Here's how the part is built. I have some questions about the finished solid (model axes, mm). Round coordinates to 2 decimals unless told otherwise and drop trailing zeros. Write each loop counter-clockwise with the first axis right and the second up, starting at its lowest first coordinate (ties: lowest second). Pieces come first, ordered by that corner, then holes. Notation, with made-up numbers: (30.25, 56.25) -> (81.25, 56.25) arc R32 ccw to (81.25, 86.25) -> close; hole circle Ø5 at (6.5, 57.25). An arc over 180 degrees is marked (long way). Answer as CSV lines item,"result".
from build123d import *

# Parameters (mm, degrees)
SKETCH001_W      = 8.45
SKETCH001_H      = 8.45
EXTRUDE001_DEPTH = 3
SKETCH_W         = 148.3
SKETCH_H         = 12.45
SKETCH_W_2       = 8.45
SKETCH_H_2       = 8.45
EXTRUDE_DEPTH    = 6.8


with BuildPart() as extrude001:
    # Sketch001 → Extrude001 (new body)
    with BuildSketch(Plane.XY):
        with Locations((-142.725, 0)):
            Rectangle(SKETCH001_W, SKETCH001_H)
        with Locations((7.5, 0)):
            Rectangle(SKETCH001_W, SKETCH001_H)
    extrude(amount=EXTRUDE001_DEPTH)


with BuildPart() as cut:
    # Sketch → Extrude (new body)
    with BuildSketch(Plane.XY):
        with Locations((-67.925, 0)):
            Rectangle(SKETCH_W, SKETCH_H)
        Rectangle(SKETCH_W_2, SKETCH_H_2, mode=Mode.SUBTRACT)
        with Locations((-10.45, 0)):
            Rectangle(SKETCH_W_2, SKETCH_H_2, mode=Mode.SUBTRACT)
        with Locations((-20.9, 0)):
            Rectangle(SKETCH_W_2, SKETCH_H_2, mode=Mode.SUBTRACT)
        with Locations((-31.35, 0)):
            Rectangle(SKETCH_W_2, SKETCH_H_2, mode=Mode.SUBTRACT)
        with Locations((-41.8, 0)):
            Rectangle(SKETCH_W_2, SKETCH_H_2, mode=Mode.SUBTRACT)
        with Locations((-52.25, 0)):
            Rectangle(SKETCH_W_2, SKETCH_H_2, mode=Mode.SUBTRACT)
        with Locations((-62.7, 0)):
            Rectangle(SKETCH_W_2, SKETCH_H_2, mode=Mode.SUBTRACT)
        with Locations((-73.15, 0)):
            Rectangle(SKETCH_W_2, SKETCH_H_2, mode=Mode.SUBTRACT)
        with Locations((-83.6, 0)):
            Rectangle(SKETCH_W_2, SKETCH_H_2, mode=Mode.SUBTRACT)
        with Locations((-94.05, 0)):
            Rectangle(SKETCH_W_2, SKETCH_H_2, mode=Mode.SUBTRACT)
        with Locations((-104.5, 0)):
            Rectangle(SKETCH_W_2, SKETCH_H_2, mode=Mode.SUBTRACT)
        with Locations((-114.95, 0)):
            Rectangle(SKETCH_W_2, SKETCH_H_2, mode=Mode.SUBTRACT)
        with Locations((-125.4, 0)):
            Rectangle(SKETCH_W_2, SKETCH_H_2, mode=Mode.SUBTRACT)
        with Locations((-135.85, 0)):
            Rectangle(SKETCH_W_2, SKETCH_H_2, mode=Mode.SUBTRACT)
    extrude(amount=EXTRUDE_DEPTH)

    # Cut: cut Extrude001
    add(extrude001.part, mode=Mode.SUBTRACT)


solid = cut.part
Item 1: I need wall thicknesses on L1, parallel to Y at x = -103.5, z = 5.5 (3 decimals). Which ranges of the line are inside material? Lowest first, please.
Results found:
L1,"y = -6.225 to -4.225, 4.225 to 6.225"
Item 2: Suppose I cut it at B-B, the plane y = -0.5. State how many separate pieces and enclosed holes the cut face has, then the cut area to 3 significant figures.
Results found:
separate pieces,"15"
enclosed holes,"0"
area,"192 mm²"
Item 3: Suppose I cut it at A-A, the plane x = -43.5. List the corners of the cut face in (y, z) for me (3 decimals).
Results found:
outline,"(-6.225, 0) -> (-4.225, 0) -> (-4.225, 6.8) -> (-6.225, 6.8) -> close; (4.225, 0) -> (6.225, 0) -> (6.225, 6.8) -> (4.225, 6.8) -> close"
Item 4: If we mould it in two halves opening along Y, with no side actions, what happens to faces 1 (the flat face through (6.225, 0, 4)), 2 (the flat face through (-137, 4.225, 3))? For each: pulls with the +Y half, pulls with the -Y half, needs draft (parallel to the pull), parting line crosses it, or undercut.
Results found:
face 1,"needs draft"
face 2,"undercut"
